Source: CAD feature listing. Evaluate the final solid. Frame: model axes, mm. A direction names the side the tool comes from. Round coordinates to 2 decimals unless told otherwise and drop trailing zeros. Loops run counter-clockwise (first coordinate to the right, second up) from the corner with the lowest first, then second, coordinate; pieces in that order, holes last. Notation, with made-up numbers: (20.5, 60) -> (68.5, 60) arc R5 cw to (68.5, 68) -> close; hole circle Ø2 at (66, -13). An arc over 180 degrees is marked (long way). Return JSON: item names as keys, results as strings. Group by question number.
```python
from build123d import *

# Parameters (mm, degrees)
F2_SIZE  = 3
F3_SIZE  = 0.5
F5_D     = 5
F7_D     = 4
F7_DEPTH = 12
F7_TIP   = 1.2017212381


with BuildPart() as f1:
    # F0 (on Front) → F1 (revolve)
    with BuildSketch(Plane.XZ):
        Polygon((0, 87.5), (0, 14.25), (5, 14.25), (5, 82.5), (40, 82.5), (40, 87.5), align=None)
    revolve(axis=Axis((15.7068069821, 0, 0), (1, 0, 0)))

    # F2
    f2_edges = [f1.edges().sort_by_distance(p)[0] for p in [
        (0, 0, -87.5),
    ]]
    chamfer(f2_edges, length=F2_SIZE)

    # F3
    f3_edges = [f1.edges().sort_by_distance(p)[0] for p in [
        (40, 0, -87.5),
        (40, 0, -82.5),
        (5, 0, -14.25),
        (0, 0, -14.25),
    ]]
    chamfer(f3_edges, length=F3_SIZE)

    # F5 (through all)
    with Locations(Plane(origin=(0, 0, 0), x_dir=(0, -1, 0), z_dir=(-1, 0, 0))):
        with Locations((0, 28), (-28, 0), (0, -28), (28, 0)):
            Hole(F5_D / 2)

    # F7
    with Locations(Plane.YZ.offset(40)):
        with Locations((0, 85), (-85, 0), (-60.1040764009, 60.1040764009), (-60.1040764009, -60.1040764009), (0, -85), (60.1040764009, -60.1040764009), (85, 0), (60.1040764009, 60.1040764009)):
            Hole(F7_D / 2, depth=F7_DEPTH)
            with Locations((0, 0, -(F7_DEPTH + F7_TIP / 2))):  # 118° drill point
                Cone(0, F7_D / 2, F7_TIP, mode=Mode.SUBTRACT)


solid = f1.part
```
(1) Cut plane A-A (x = 34). Count the separate pieces of the cut face and the enclosed holes in it, and give its area (3 significant figures).
(2) Cut plane B-B (x = 21). Return loops of the section in (y, z).
(3) Mould query, pull axis Z, two halves, no side actions, for faces 1 (the face through (40, 77, 33)), 2 (the face through (2.53, -0.33, -25.52)), 3 (the face through (34, 0, -83)). Classes: released by +Z, released by -Z, zero draft, split by the parting line, or undercut.
(4) Pin query (flat end, axial travel): pin 1 (4 mm diameter, centred on x = 20, z = 48, fed in from -Y); pin 2 (6 mm diameter, centred on y = -20, z = 24.5, fed in from +X); pin 3 (6 mm diameter, centred on x = 7.5, z = -32, fed in from +Y); pin 4 (3 mm diameter, centred on y = -28, z = 0, fed in from -X). Return the tip coordinate at first contact, or that it passes through.
(5) Set-up query: faces 4 (the face through (5, 17, 1)), 5 (the face through (2.528, 5.458, 13.163)). Return all of +Z, -Z, +X, -X, +Y, -Y with unobstructed straight access to the full face (end or side cutting, diameter ignored); none if empty.
(6) Ray query, line 1 (Y direction, x = 37.5, z = 0); line 2 (Y direction, x = 35.5, z = 59). Return the intervals inside material, ascending.
Answers follow:
{
 "1": {"separate pieces": "1", "enclosed holes": "9", "area": "2,570 mm^2"},
 "2": {"outline": "circle Ø175 at (0, 0); hole circle Ø165 at (0, 0)"},
 "3": {"face 1": "zero draft", "face 2": "undercut", "face 3": "undercut"},
 "4": {"pin 1": "y = -74.43", "pin 2": "x = 5", "pin 3": "y = 82.55", "pin 4": "through"},
 "5": {"face 4": "+X", "face 5": "+X, -X"},
 "6": {"line 1": "-87.5 to -87, -83 to -82.5, 82.5 to 83, 87 to 87.5", "line 2": "-64.62 to -61.77, -58.44 to -57.66, 57.66 to 58.44, 61.77 to 64.62"}
}
